from build123d import *

# Parameters (mm, degrees)
FILLET_1_R = 0.5


with BuildPart() as part:
    # 草图1 → 旋转1 (revolve)
    with BuildSketch(Plane.XY, mode=Mode.PRIVATE) as revolve_1_sk:
        Polygon((0, 2), (-3, 2), (-3, 6.5), (-2, 6.5), (0, 4.5), align=None)
    revolve_1 = revolve(revolve_1_sk.sketch.rotate(Axis((-66.431667693, 0, 0), (1, 0, 0)), 90), axis=Axis((-66.431667693, 0, 0), (1, 0, 0)))

    # 镜向1: 旋转1 across plane
    add(revolve_1.mirror(Plane(origin=(0, 0, 0), x_dir=(0, 0, 1), z_dir=(1, 0, 0))))

    # 圆角1
    fillet_1_edges = [part.edges().sort_by_distance(p)[0] for p in [
        (0, 0, -4.5),
    ]]
    fillet(fillet_1_edges, radius=FILLET_1_R)


solid = part.part
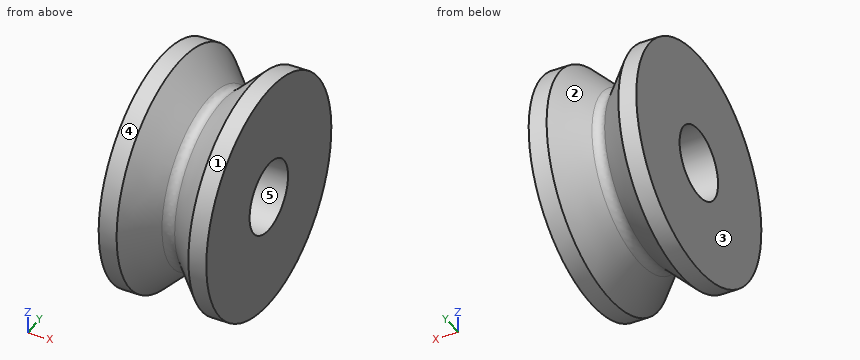
Verification items for the finished model (mm, model axes). Face numbers are marked on the shaded views. A direction names the side the tool comes from. Round coordinates to 2 decimals unless told otherwise and drop trailing zeros. Loops run counter-clockwise (first coordinate to the right, second up) from the corner with the lowest first, then second, coordinate; pieces in that order, holes last. Notation, with made-up numbers: (1.5, 0.25) - (23.5, 0.25) arc R20 cw to (23.5, 30.25) - close; hole circle Ø3 at (-7.75, 67). An arc over 180 degrees is marked (long way). Use one line per item in the form item = value.
1. Draft check along Y on the marked faces 3, 4 and 5. Enter one of: pulls with the +Y half, pulls with the -Y half, needs draft (parallel to the pull), parting line crosses it, or undercut.
A:
face_3 = needs draft
face_4 = parting line crosses it
face_5 = undercut
2. Section check A-A on x = -2.55. Record the cut outline in (y, z).
A:
outline = circle Ø13 at (0, 0); hole circle Ø4 at (0, 0)
3. Gauge pin test, flat ends, axial feed: pin 1 Ø3 at (x, z) = (-1, -3.5) entering from +Y; pin 2 Ø2.5 at (y, z) = (0, 0) entering from -X. Record the tip position at first contact, or that the pin passes through.
A:
pin_1 = 6.05
pin_2 = through
4. Access from +Z, -Z, +X, -X, +Y, -Y to the whole of each face (thin tool, end or side, straight path). Record for the marked faces 1 and 2.
A:
face_1 = +X, -X
face_2 = none
5. Scan lines: probe 1 along Z at (x, y) = (-0.1, -1.5); probe 2 along X at (y, z) = (3.75, 3.25); probe 3 along Y at (x, z) = (1.2, 0). Record each from-to range of solid material in increasing order.
A:
probe_1 = -4.47 to -1.32, 1.32 to 4.47
probe_2 = -3 to -0.46, 0.46 to 3
probe_3 = -5.7 to -2, 2 to 5.7
